The listing builds one solid part. Answer for the finished solid, in the listing's coordinates (mm). A direction names the side the tool comes from. Give positions to 0.01 mm unless a question says otherwise; leave off trailing zeros. Order: outer loops, then holes, each group sorted by start corner. A loop starts at its lowest first (then second) coordinate and runs counter-clockwise, first axis right, second up. Notation, with made-up numbers: (63.25, 50.25) - (104.25, 50.25) arc R9 cw to (104.25, 66.25) - close; hole circle Ø1 at (-17, 65). An arc over 180 degrees is marked (long way). Answer as a JSON object with one key per item and string values. Group by question number.
Q1. Consider line 1 (Z direction, x = -10, y = -7); line 2 (Z direction, x = -26, y = -8.25); line 3 (X direction, y = -8, z = -19.5). Determine where each line is inside the solid, lowest interval first.
Q2. Given pin 1 (1.6 mm diameter, centred on x = -56, z = -51.5, fed in from +Y); pin 2 (8 mm diameter, centred on x = -14.5, z = -9, fed in from -Y); pin 3 (6 mm diameter, centred on y = 1.5, z = -24, fed in from -X), each flat-ended and moving along its own axis, determine where each tip first touches the part or whether it passes through.
Q3. The mould has two halves that part along Y. Classify faces 4 (the face through (-28, 1, 50)), 5 (the face through (-58, 0, -50)), 6 (the face through (-57, 10, 51.2)): released by +Y, released by -Y, zero draft, split by the parting line, or undercut.
Q4. A cutting plane is placed at B-B, the plane y = 0. Give the vertices of the cut face in (x, z), and give its area (3 significant figures).
Q5. A cutting plane is placed at A-A, the plane x = -21. Give the vertices of the cut face in (y, z).
Q6. A cutting plane is placed at C-C, the plane z = 39.5. Give the vertices of the cut face in (x, y).
Q7. For faces 1 (the face through (-28, -8, -49)), 2 (the face through (-56, 0, -51)), 3 (the face through (-28, -9, 47)), determine the directions among +Z, -Z, +X, -X, +Y, -Y from which every point of the face is accessible in a straight line to the end or side of a thin tool.
Autodesk Inventor part; units mm, degrees
ref_plane "YZ Plane" through (0, 0, 0) normal (1, 0, 0) x (0, 1, 0)
ref_plane "XZ Plane" through (0, 0, 0) normal (0, 1, 0) x (-1, 0, 0)
ref_plane "XY Plane" through (0, 0, 0) normal (0, 0, 1) x (1, 0, 0)
sketch "Sketch1" plane through (0, 0, 0) normal (1, 0, 0) x (0, 1, 0)
  line L0 (10, 52) -> (-10, 52)
  line L1 (-10, 52) -> (-10, -52)
  line L2 (-10, -52) -> (10, -52)
  line L3 (10, -52) -> (10, 52)
  point P0 (0, 0)
  dimension "d0" = 104
  dimension "d1" = 20
  dimension "d2" = 52
  dimension "d3" = 10
extrude "Extrusion1" add sketch "Sketch1" against normal blind 2
sketch "Sketch2" plane through (-2, 0, 0) normal (-1, 0, 0) x (0, 0, 1)
  line L0 (52, 10) -> (-52, 10)
  line L1 (-52, -10) -> (52, -10)
  line L2 (-52, 10) -> (-50, 10)
  line L3 (-50, 10) -> (-50, -10)
  line L4 (-50, -10) -> (-52, -10)
  line L5 (-52, -10) -> (-52, 10)
  line L6 (52, -10) -> (52, 10)
  line L7 (52, 10) -> (50, 10)
  line L8 (50, 10) -> (50, -10)
  line L9 (50, -10) -> (52, -10)
  line L10 (52, -10) -> (52, 10)
  point P0 (0, 0)
  dimension "d6" = 2
  dimension "d7" = 2
extrude "Extrusion2" add sketch "Sketch2" along normal blind 57 contours L6 L1 L8 L0 | L3 L1 L5 L0
sketch "Sketch3" plane through (0, 0, 0) normal (1, 0, 0) x (0, 0, -1)
  line L0 (52, 10) -> (-52, 10)
  line L1 (52, 10) -> (-52, 10)
  line L2 (-52, 10) -> (-52, 12)
  line L3 (-52, 12) -> (52, 12)
  line L4 (52, 12) -> (52, 10)
  line L5 (-52, 10) -> (-52, -10)
  point P0 (0, 0)
  dimension "d10" = 2
  dimension "d11" = 0
extrude "Extrusion3" add sketch "Sketch3" against normal blind 54
sketch "Sketch6" plane through (-2, -10, 50) normal (0, 0, -1) x (-1, 0, 0)
  line L0 (52, 20) -> (57, 20)
  line L1 (0, 0) -> (57, 0)
  line L2 (52, 20) -> (55, 20)
  line L3 (55, 20) -> (55, 0)
  line L4 (55, 0) -> (52, 0)
  line L5 (52, 0) -> (52, 20)
  line L6 (57, 20) -> (57, 0)
  point P0 (-2, 10)
  dimension "d16" = 2
  dimension "d17" = 3
sketch "Sketch7" plane through (-59, -10, -50) normal (0, 0, 1) x (1, 0, 0)
  line L0 (5, 20) -> (0, 20)
  line L1 (59, 0) -> (0, 0)
  line L2 (2, 20) -> (5, 20)
  line L3 (5, 20) -> (5, 0)
  line L4 (5, 0) -> (2, 0)
  line L5 (2, 0) -> (2, 20)
  line L6 (0, 0) -> (0, 20)
  point P0 (59, 10)
  dimension "d18" = 3
  dimension "d19" = 2
extrude "Extrusion4" cut sketch "Sketch7" against normal blind 1 contours L3 L1 L5 L0
extrude "Extrusion5" cut sketch "Sketch6" against normal blind 1 contours L0 L3 L1 L5
sketch "Sketch8" plane through (-2, -10, -50) normal (0, 0, 1) x (1, 0, 0)
  line L0 (-52, 20) -> (-52, 0)
  line L1 (0, 0) -> (-52, 0)
  line L2 (-52, 0) -> (-52, 2)
  line L3 (-52, 2) -> (0, 2)
  line L4 (0, 2) -> (0, 0)
  point P0 (2, 10)
  dimension "d24" = 2
sketch "Sketch9" plane through (-2, -10, 50) normal (0, 0, -1) x (-1, 0, 0)
  line L0 (52, 0) -> (0, 0)
  line L1 (0, 0) -> (0, 2)
  line L2 (0, 2) -> (52, 2)
  line L3 (52, 2) -> (52, 0)
  point P0 (-2, 10)
  dimension "d25" = 2
extrude "Extrusion6" add sketch "Sketch8" along normal blind 3
extrude "Extrusion7" add sketch "Sketch9" along normal blind 3
properties part number "LEDs_protect"
Reply:
{
 "1": {"line 1": "z = -52 to -50, 50 to 52", "line 2": "z = -52 to -47, 47 to 52", "line 3": "x = -2 to 0"},
 "2": {"pin 1": "stops at y = 10", "pin 2": "stops at y = 10", "pin 3": "stops at x = -2"},
 "3": {"face 4": "undercut", "face 5": "zero draft", "face 6": "released by +Y"},
 "4": {"outline": "(-59, -52) - (0, -52) - (0, 52) - (-59, 52) - (-59, 50) - (-57, 50) - (-57, 51) - (-54, 51) - (-54, 50) - (-2, 50) - (-2, -50) - (-54, -50) - (-54, -51) - (-57, -51) - (-57, -50) - (-59, -50) - close", "area": "430 mm^2"},
 "5": {"outline": "(-10, -52) - (12, -52) - (12, 52) - (-10, 52) - (-10, 47) - (-8, 47) - (-8, 50) - (10, 50) - (10, -50) - (-8, -50) - (-8, -47) - (-10, -47) - close"},
 "6": {"outline": "(-54, 10) - (-2, 10) - (-2, -10) - (0, -10) - (0, 12) - (-54, 12) - close"},
 "7": {"face 1": "-X", "face 2": "+Y, -Y", "face 3": "-X, -Y"}
}
